```python
from build123d import *

# Parameters (mm, degrees)
F0_W = 12.7
F0_H = 6.35
F2_R = 6.34999
F3_R = 6.34999


# Not quite as in the source:
# - a fillet or chamfer is up to 0.001 mm smaller than in the source, because OpenCascade refuses the exact size


with BuildPart() as f1:
    # F0 (on Top) → F1 (revolve)
    with BuildSketch(Plane.XY):
        Rectangle(F0_W, F0_H)
    revolve(axis=Axis((31.75, -0.4141320733, 0), (0, -1, 0)))

    # F2 (radius 6.35 in the source; OpenCascade refuses exactly that, so slightly less here)
    f2_edges = [f1.edges().sort_by_distance(p)[0] for p in [
        (57.15, 3.175, 0),
    ]]
    fillet(f2_edges, radius=F2_R)

    # F3 (radius 6.35 in the source; OpenCascade refuses exactly that, so slightly less here)
    f3_edges = [f1.edges().sort_by_distance(p)[0] for p in [
        (69.85, 3.175, 0),
    ]]
    fillet(f3_edges, radius=F3_R)

    # F4: F1 across plane


with BuildPart() as f1_1:
    add(f1.part)
    add(f1.part.mirror(Plane.XZ), mode=Mode.INTERSECT)


solid = f1_1.part
```
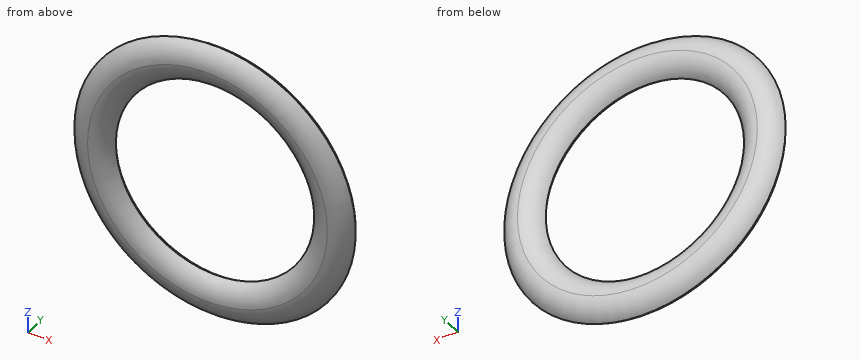
Source: CAD feature listing. Evaluate the final solid. Frame: model axes, mm. Coordinates: 2 decimals unless noted, no trailing zeros. Write each loop counter-clockwise with the first axis right and the second up, starting at its lowest first coordinate (ties: lowest second). Pieces come first, ordered by that corner, then holes. Notation, with made-up numbers: (44, -1.75) -> (50, -1.75) arc R15 ccw to (50, 4.25) -> close; hole circle Ø1 at (73.5, 58). An arc over 180 degrees is marked (long way). Return JSON: item names as keys, results as strings. Group by question number.
1) Ray query, line 1 along X through (y, z) = (1.5, 2.5); line 2 along X through (y, z) = (0.5, 2); line 3 along Z through (x, y) = (10.5, 1.5). Return the intervals inside material, ascending.
2) Contact query for flat-ended pins moving along their axis: P1, Ø12, axis at x = 48.5, z = -13.5, coming from the +Y side; P2, Ø1.5, axis at y = -2.5, z = 21, coming from the -X side; P3, Ø1, axis at y = 1, z = 12.5, coming from the -X side. Output: stop coordinate, or through.
3) Section query B-B, the plane y = -2. Return loops of the section in (x, z).
4) Section query A-A, the plane y = 2.25. Return loops of the section in (x, z).
From the geometry:
{
 "1": {"line 1": "-4.21 to 4.41, 59.09 to 67.71", "line 2": "-5.12 to 5.25, 58.25 to 68.62", "line 3": "-29.12 to -17.38, 17.38 to 29.12"},
 "2": {"P1": "y = 1.55", "P2": "x = 2.69", "P3": "x = -3.04"},
 "3": {"outline": "circle Ø70.86 at (31.75, 0); hole circle Ø56.14 at (31.75, 0)"},
 "4": {"outline": "circle Ø70.1 at (31.75, 0); hole circle Ø56.9 at (31.75, 0)"}
}
